For this review, take the finished solid that the model builds, in its own axes (mm). Face numbers are marked on the shaded views. A direction names the side the tool comes from. Round coordinates to 2 decimals unless told otherwise and drop trailing zeros. Loops run counter-clockwise (first coordinate to the right, second up) from the corner with the lowest first, then second, coordinate; pieces in that order, holes last.
1) Insertion check: pin 1 (3 mm diameter, centred on x = -2.5, z = 7, fed in from +Y); pin 2 (4 mm diameter, centred on y = -2, z = 12, fed in from -X); pin 3 (4 mm diameter, centred on x = 8.5, z = -3, fed in from -Y); pin 4 (4 mm diameter, centred on y = -4.5, z = -9.5, fed in from +X). Each pin has a flat end and moves straight along its axis. Give the tip position at first contact, or say it passes through.
2) Tool access review of the marked faces 5, 6, 7, 8 and 9: name each direction out of +Z, -Z, +X, -X, +Y, -Y from which nothing blocks a thin tool from reaching the whole face with its end or side.
3) Mouldability with a two-part tool opening along Z and no side actions: class the marked faces 1, 2, 3 and 4 as pulls with the +Z half, pulls with the -Z half, needs draft (parallel to the pull), parting line crosses it, or undercut.
4) Take a section at B-B (y = -8). State the section outline as (x, z) points.
5) Take a section at D-D (y = -5.5). State the section outline as (x, z) points, then the cut area to 3 significant figures.
6) Take a section at C-C (x = 0). State the section outline as (y, z) points, then the cut area to 3 significant figures.
7) Wall thickness on L1, parallel to Z at x = 0, y = -1.8; L2, parallel to Z at x = -3.5, y = -7.5; L3, parallel to Y at x = -3, z = 6: over which ranges is each line inside the solid? List them lowest first.
8) Take a section at A-A (z = 0). State the section outline as (x, y) points, then the cut area to 3 significant figures.
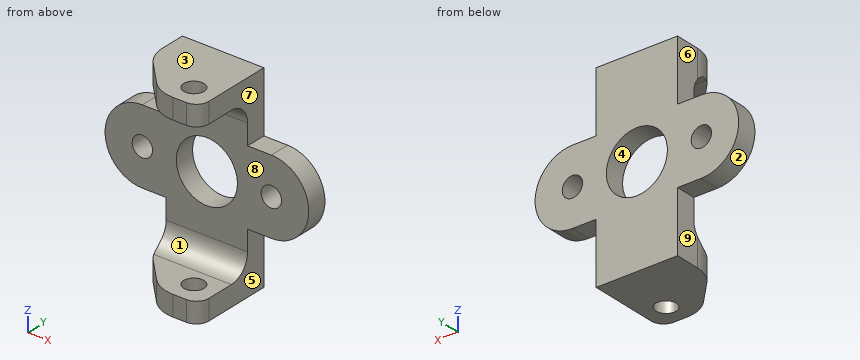
```python
from build123d import *

# Parameters (mm, degrees)
F0_R     = 1.5
F0_R_2   = 4.5
F1_DEPTH = 3
F2_W     = 12
F2_H     = 29
F3_DEPTH = 3
F4_R     = 1.5
F5_DEPTH = 3
F7_R     = 3
F8_R     = 4.5
F9_DEPTH = 3


with BuildPart() as f1:
    # F0 (on Front) → F1 (new body)
    with BuildSketch(Plane.XZ):
        with BuildLine():
            Line((0, -5.5), (9.5, -5.5))
            ThreePointArc((9.5, -5.5), (15, 0), (9.5, 5.5))
            Line((9.5, 5.5), (0, 5.5))
            Line((0, 5.5), (-9.5, 5.5))
            ThreePointArc((-9.5, 5.5), (-15, 0), (-9.5, -5.5))
            Line((-9.5, -5.5), (0, -5.5))
        make_face()
        with Locations((-9.5, 0)):
            Circle(F0_R, mode=Mode.SUBTRACT)
        Circle(F0_R_2, mode=Mode.SUBTRACT)
        with Locations((9.5, 0)):
            Circle(F0_R, mode=Mode.SUBTRACT)
    extrude(amount=F1_DEPTH)

    # F2 (on face) → F3 (join)
    with BuildSketch(Plane.XZ.offset(3)):
        Rectangle(F2_W, F2_H)
    extrude(amount=-F3_DEPTH)

    # F4 (on face) → F5 (join)
    with BuildSketch(Plane(origin=(0, 0, -14.5), x_dir=(1, 0, 0), z_dir=(0, 0, -1))):
        with BuildLine():
            Line((-6, 0), (6, 0))
            Line((6, 0), (6, 10.1512318682))
            ThreePointArc((6, 10.1512318682), (5.458508351, 11.458508351), (4.1512318682, 12))
            Line((4.1512318682, 12), (2.1505740618, 12))
            ThreePointArc((2.1505740618, 12), (0.1749902584, 11.5931545408), (-1.4790906252, 10.4388274542))
            Line((-1.4790906252, 10.4388274542), (-4.629664687, 7.11341274))
            ThreePointArc((-4.629664687, 7.11341274), (-5.6447994271, 5.5254873044), (-6, 3.6745852858))
            Line((-6, 3.6745852858), (-6, 0))
        make_face()
        with Locations((2.5998784695, 8.662102744)):
            Circle(F4_R, mode=Mode.SUBTRACT)
    extrude(amount=-F5_DEPTH)

    # F6: F1 across plane


with BuildPart() as f1_1:
    add(f1.part)
    add(f1.part.mirror(Plane.XY))

    # F7
    f7_edges = [f1_1.edges().sort_by_distance(p)[0] for p in [
        (0, -3, 11.5),
        (0, -3, -11.5),
    ]]
    fillet(f7_edges, radius=F7_R)

    # F8 (on face) → F9 (cut, through all)
    with BuildSketch(Plane(origin=(0, 0, 0), x_dir=(-1, 0, 0), z_dir=(0, 1, 0))):
        Circle(F8_R)
    extrude(amount=-F9_DEPTH, mode=Mode.SUBTRACT)


solid = f1_1.part
```
Response:
1. pin 1: stops at y = 0
1. pin 2: stops at x = -6
1. pin 3: stops at y = -3
1. pin 4: stops at x = 6
2. face 5: -Z, +X, +Y, -Y
2. face 6: +Z, -X, +Y, -Y
2. face 7: +Z, +X, +Y, -Y
2. face 8: +X, -X, -Y
2. face 9: -Z, -X, +Y, -Y
3. face 1: undercut
3. face 2: parting line crosses it
3. face 3: pulls with the +Z half
3. face 4: undercut
4. outline: (-3.79, -14.5) - (1.25, -14.5) - (1.25, -11.5) - (-3.79, -11.5) - close; (-3.79, 11.5) - (1.25, 11.5) - (1.25, 14.5) - (-3.79, 14.5) - close; (3.95, -14.5) - (6, -14.5) - (6, -11.5) - (3.95, -11.5) - close; (3.95, 11.5) - (6, 11.5) - (6, 14.5) - (3.95, 14.5) - close
5. outline: (-5.65, -14.5) - (6, -14.5) - (6, -11.46) - (-5.65, -11.46) - close; (-5.65, 11.46) - (6, 11.46) - (6, 14.5) - (-5.65, 14.5) - close
5. area: 70.9 mm2
6. outline: (-11.51, -14.5) - (0, -14.5) - (0, -4.5) - (-3, -4.5) - (-3, -8.5) arc R3 cw to (-6, -11.5) - (-11.51, -11.5) - close; (-11.51, 11.5) - (-6, 11.5) arc R3 cw to (-3, 8.5) - (-3, 4.5) - (0, 4.5) - (0, 14.5) - (-11.51, 14.5) - close
6. area: 115 mm2
7. L1: z = -14.5 to -4.5, 4.5 to 14.5
7. L2: z = -14.5 to -11.5, 11.5 to 14.5
7. L3: y = -3 to 0
8. outline: (-15, -3) - (-11, -3) - (-11, 0) - (-15, 0) - close; (-8, -3) - (-4.5, -3) - (-4.5, 0) - (-8, 0) - close; (4.5, -3) - (8, -3) - (8, 0) - (4.5, 0) - close; (11, -3) - (15, -3) - (15, 0) - (11, 0) - close
8. area: 45.0 mm2
